Verification items for the finished model (mm, model axes). Face numbers are marked on the shaded views. A direction names the side the tool comes from. Coordinates: 2 decimals unless noted, no trailing zeros. Loops run counter-clockwise (first coordinate to the right, second up) from the corner with the lowest first, then second, coordinate; pieces in that order, holes last. Notation, with made-up numbers: (7.25, 36) - (47.25, 36) arc R24 cw to (47.25, 52) - close; hole circle Ø4 at (-12.5, -16). An arc over 180 degrees is marked (long way). One line per item, written item: value. Start each with the question number.
(1) Draft check along X on the marked faces 1, 2, 3 and 4. Enter one of: +X half, -X half, draft (parallel to the pull), parting line (faces both ways), or undercut.
(2) Section check C-C (y = 2.5). Record the boundary of the cut face in (x, z), plus the area to 3 significant figures.
(3) Thickness scan on probe 1 along X at (y, z) = (6, -33); probe 2 along Z at (x, y) = (-5.75, 6); probe 3 along X at (y, z) = (3.75, -13). Record the ranges inside material, lowest first. Write a range as [from, to].
(4) Section check D-D (x = -4.5). Record the boundary of the cut face in (y, z).
(5) Set-up check for the marked faces 5, 6, 7 and 8: record each of +Z, -Z, +X, -X, +Y, -Y from which the full face is reachable in a straight line by a thin tool's end or side.
(6) Gauge pin test, flat end, axial feed: P1, Ø4.5, axis at y = 6, z = -25, coming from the +X side. Record the tip position at first contact, or that the pin passes through.
(7) Section check B-B (z = -17). Record the boundary of the cut face in (x, y).
(8) Section check A-A (y = 6). Record the boundary of the cut face in (x, z), plus the area to 3 significant figures.
Autodesk Inventor part; units mm, degrees
ref_plane "YZ Plane" through (0, 0, 0) normal (1, 0, 0) x (0, 1, 0)
ref_plane "XZ Plane" through (0, 0, 0) normal (0, 1, 0) x (-1, 0, 0)
ref_plane "XY Plane" through (0, 0, 0) normal (0, 0, 1) x (1, 0, 0)
sketch "Esboço1" plane through (0, 0, 0) normal (0, 1, 0) x (-1, 0, 0)
  line L0 (0, 0) -> (45.5, 0)
  line L1 (45.5, 0) -> (45.5, -35.75)
  line L2 (49.75, -40) -> (49.75, -40)
  line L3 (54, -35.75) -> (54, 0)
  line L4 (54, 0) -> (64, 0)
  line L5 (64, 0) -> (64, -50)
  line L6 (64, -50) -> (18.5, -50)
  line L7 (18.5, -50) -> (18.5, -14.25)
  line L8 (14.25, -10) -> (14.25, -10)
  line L9 (10, -14.25) -> (10, -50)
  line L10 (10, -50) -> (0, -50)
  line L11 (0, -50) -> (0, 0)
  arc A0 (18.5, -14.25) -> (14.25, -10) centre (14.25, -14.25) ccw
  arc A1 (14.25, -10) -> (10, -14.25) centre (14.25, -14.25) ccw
  arc A2 (45.5, -35.75) -> (49.75, -40) centre (49.75, -35.75) ccw
  arc A3 (49.75, -40) -> (54, -35.75) centre (49.75, -35.75) ccw
  point P0 (45.5, -40)
  point P1 (54, -40)
  point P2 (10, -10)
  dimension "d0" = 64
  dimension "d1" = 10
  dimension "d2" = 40
  dimension "d3" = 50
  dimension "d4" = 8.5
  dimension "d5" = 4.25
extrude "Extrusão1" add sketch "Esboço1" along normal blind 12
sketch "Esboço2" plane through (0, 0, 0) normal (1, 0, 0) x (0, 0, -1)
  line L0 (0, 12) -> (50, 12)
  line L1 (50, 0) -> (50, 12)
  point P0 (0, 0)
  point P1 (25, 6)
  dimension "d8" = 50
  dimension "d9" = 12
  dimension "d10" = 6
  dimension "d11" = 25
hole "Furo1" at (0, 6, -25) direction (-1, 0, 0) diameter 4.917 depth 10
sketch "Esboço3" plane through (-64, 0, -50) normal (-1, 0, 0) x (0, 0, 1)
  line L0 (0, 0) -> (50, 0)
  line L1 (0, 0) -> (0, 12)
  circle A0 centre (25, 6) radius 2.4585
  dimension "d19" = 50
  dimension "d20" = 12
hole "Furo2" at (-64, 6, -25) direction (1, 0, 0) diameter 4.917 depth 10
sketch "Sketch4" plane through (0, 12, 0) normal (0, 1, 0) x (1, 0, 0)
  line L0 (-36.5, 10) -> (-27.4995, 10)
  arc A0 (-27.4995, 10) -> (-27.4995, 24) centre (-27.4995, 17) ccw
  arc A1 (-36.5002, 24) -> (-36.5, 10) centre (-36.5, 17) ccw
  line L1 (-36.5, 24) -> (-27.4995, 24)
  line L2 (-13.5, 10) -> (-19.5, 10)
  line L3 (-36.5002, 26.001) -> (-27.4998, 26.001)
  arc A2 (-27.4998, 26.001) -> (-27.6165, 40) centre (-27.4998, 33.001) ccw
  arc A3 (-36.6169, 40) -> (-36.5002, 26.001) centre (-36.5002, 33.001) ccw
  line L4 (-36.6169, 40) -> (-27.6165, 40)
  line L5 (-45.5, 35.75) -> (-45.5, 0)
  line L6 (-50.5, 40) -> (-44.5, 40)
  line L7 (-18.5, 14.25) -> (-18.5, 50)
  line L8 (-36.5002, 26.001) -> (-27.4995, 26.001)
  line L9 (-27.4995, 26.001) -> (-27.4995, 24)
  line L10 (-27.4995, 24) -> (-36.5002, 24)
  line L11 (-36.5002, 24) -> (-36.5002, 26.001)
  point P0 (0, 0)
  point P1 (-31.9998, 10)
  point P2 (-20.5, 33.0593)
  point P3 (-43.5, 32.9426)
  point P4 (-32, 26.001)
  point P5 (-43.5, 16.9999)
  dimension "d28" = 0
  dimension "d29" = 0
  dimension "d30" = 23
  dimension "d31" = 13.5
  dimension "d32" = 27
  dimension "d33" = 0
  dimension "d34" = 7
  dimension "d35" = 0
extrude "Extrusion2" cut sketch "Sketch4" against normal through all
equation "\"d17\" = Espessura"
equation "\"Raio_vergadura\" = Espessura"
equation "\"Largura_alívio_de_vergadura\" = Espessura"
equation "\"Profundidade_alívio_de_vergadura\" = 0.5 * Espessura"
equation "\"Tamanho_alívio_de_dobra\" = 4 * Espessura"
equation "\"Remanescente_mínimo\" = 2 * Espessura"
equation "\"Raiodetransição\" = Raio_vergadura"
equation "\"Tamanho_de_raio_de_Jacobi\" = Raio_vergadura"
equation "\"TamanhoFolga\" = Espessura"
properties part number "Célula de carga" material "Alumínio 6061"
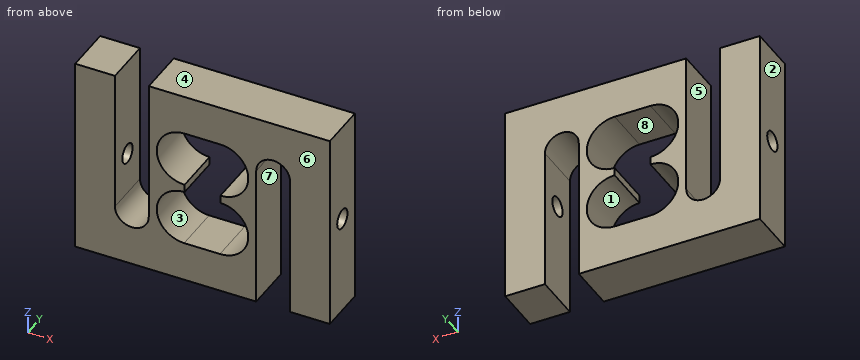
Responses:
1. face 1: undercut
1. face 2: -X half
1. face 3: undercut
1. face 4: draft
2. outline: (-64, -50) - (-18.5, -50) - (-18.5, -14.25) arc R4.25 cw to (-10, -14.25) - (-10, -50) - (0, -50) - (0, 0) - (-45.5, 0) - (-45.5, -35.75) arc R4.25 cw to (-54, -35.75) - (-54, 0) - (-64, 0) - close; hole (-36.62, -40) - (-27.62, -40) arc R7 ccw (long way) to (-27.5, -26) - (-27.5, -24) arc R7 ccw to (-27.5, -10) - (-36.5, -10) arc R7 ccw to (-36.5, -24) - (-36.5, -26) arc R7 ccw to start
2. area: 1,960 mm²
3. probe 1: x = [-64, -54], [-45.5, -43.5], [-20.5, -18.5], [-10, 0]
3. probe 2: z = [-50, -27.46], [-22.54, 0]
3. probe 3: x = [-64, -54], [-45.5, -42.24], [-21.75, -18.31], [-10.19, 0]
4. outline: (0, -50) - (12, -50) - (12, 0) - (0, 0) - close; hole circle Ø4.92 at (6, -25)
5. face 5: +Z, +Y, -Y
5. face 6: +Z, -Z, +X, -X, -Y
5. face 7: -Z, +Y, -Y
5. face 8: +Y, -Y
6. P1: stops at x = -18.5
7. outline: (-64, 0) - (-54, 0) - (-54, 12) - (-64, 12) - close; (-45.5, 0) - (-43.5, 0) - (-43.5, 12) - (-45.5, 12) - close; (-20.5, 0) - (-18.5, 0) - (-18.5, 12) - (-20.5, 12) - close; (-10, 0) - (0, 0) - (0, 12) - (-10, 12) - close
8. outline: (-64, -50) - (-18.5, -50) - (-18.5, -14.25) arc R4.25 cw to (-10, -14.25) - (-10, -22.54) - (0, -22.54) - (0, 0) - (-45.5, 0) - (-45.5, -35.75) arc R4.25 cw to (-54, -35.75) - (-54, -27.46) - (-64, -27.46) - close; (-64, -22.54) - (-54, -22.54) - (-54, 0) - (-64, 0) - close; (-10, -50) - (0, -50) - (0, -27.46) - (-10, -27.46) - close; hole (-36.62, -40) - (-27.62, -40) arc R7 ccw (long way) to (-27.5, -26) - (-27.5, -24) arc R7 ccw to (-27.5, -10) - (-36.5, -10) arc R7 ccw to (-36.5, -24) - (-36.5, -26) arc R7 ccw to start
8. area: 1,860 mm²
